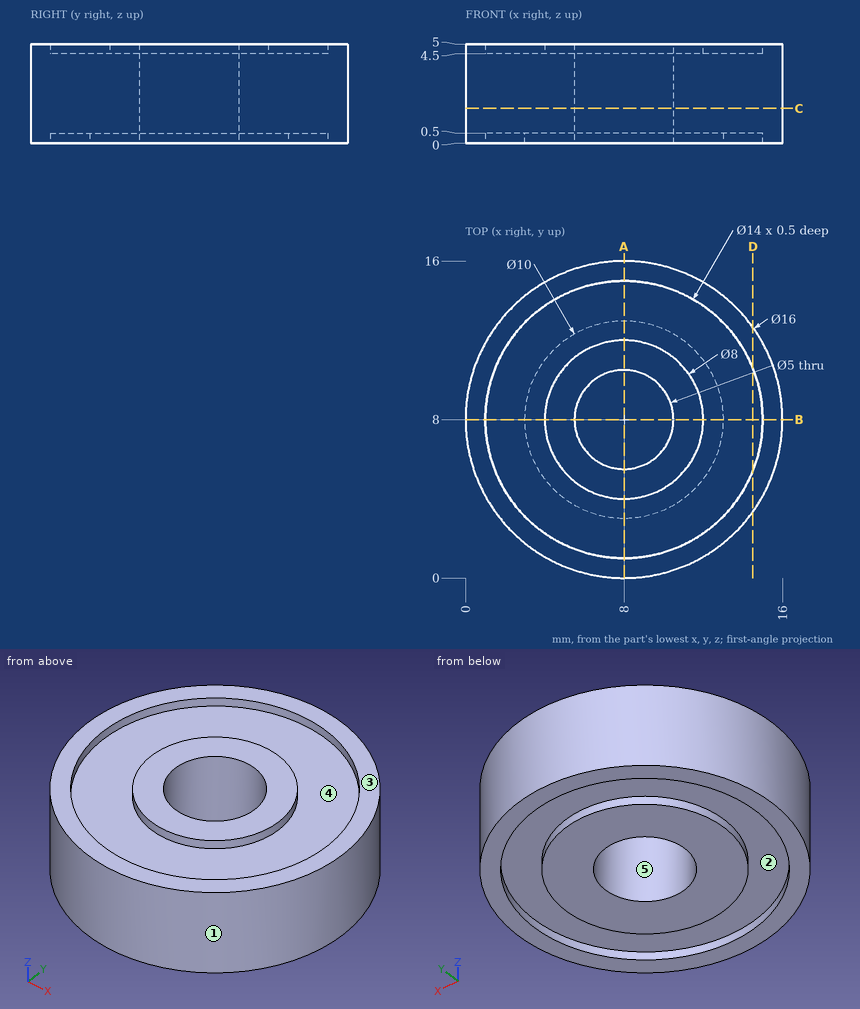
Verification items for this drawing (mm, ordinates from the low corner). A direction names the side the tool comes from. Give positions to 0.01 mm unless a question says otherwise; leave off trailing zeros. Loops run counter-clockwise (first coordinate to the right, second up) from the corner with the lowest first, then second, coordinate; pieces in that order, holes last. Notation, with made-up numbers: M 34,84.25 L 72,84.25 A19 cw 72,108.25 Z; hole C -3,67.5 d1. An arc over 180 degrees is marked long. Answer as a JSON object with one key per item and string values. Group by question number.
Item 1: Access from +Z, -Z, +X, -X, +Y, -Y to the whole of each face (thin tool, end or side, straight path). Record for the marked faces 4 and 5.
Item 2: Material ranges on L1, parallel to Y at x = 8, z = 4.85; L2, parallel to Y at x = 8, z = 0.4; L3, parallel to X at y = 8.25, z = 1.1, recorded low to high.
Item 3: Gauge pin test, flat end, axial feed: pin 1 (2 mm diameter, centred on y = 12.5, z = 3.5, fed in from -X). Record the tip position at first contact, or that the pin passes through.
Item 4: Sectioned sample at D-D on x = 14.5. Record the boundary of the cut face in (y, z), plus the area to 3 significant figures.
Item 5: Mould release check, pull along Y, two halves, no side actions. Record for the marked faces 1, 2 and 3: pulls with the +Y half, pulls with the -Y half, needs draft (parallel to the pull), parting line crosses it, or undercut.
Item 6: Sectioned sample at A-A on x = 8. Record the boundary of the cut face in (y, z), plus the area to 3 significant figures.
Item 7: Sectioned sample at C-C on z = 1.75. Record the boundary of the cut face in (x, y), plus the area to 3 significant figures.
Findings below:
{
 "1": {"face 4": "+Z", "face 5": "+Z, -Z"},
 "2": {"L1": "0 to 1, 4 to 5.5, 10.5 to 12, 15 to 16", "L2": "0 to 1, 3 to 5.5, 10.5 to 13, 15 to 16", "L3": "0 to 5.51, 10.49 to 16"},
 "3": {"pin 1": "x = 0.81"},
 "4": {"outline": "M 3.34,0 L 5.4,0 L 5.4,0.5 L 10.6,0.5 L 10.6,0 L 12.66,0 L 12.66,5 L 10.6,5 L 10.6,4.5 L 5.4,4.5 L 5.4,5 L 3.34,5 Z", "area": "41.4 mm2"},
 "5": {"face 1": "parting line crosses it", "face 2": "undercut", "face 3": "needs draft"},
 "6": {"outline": "M 0,0 L 1,0 L 1,0.5 L 3,0.5 L 3,0 L 5.5,0 L 5.5,5 L 4,5 L 4,4.5 L 1,4.5 L 1,5 L 0,5 Z; M 10.5,0 L 13,0 L 13,0.5 L 15,0.5 L 15,0 L 16,0 L 16,5 L 15,5 L 15,4.5 L 12,4.5 L 12,5 L 10.5,5 Z", "area": "50.0 mm2"},
 "7": {"outline": "C 8,8 d16; hole C 8,8 d5", "area": "181 mm2"}
}
